The figure shows three views and two pictorial views of one solid part (mm, origin at its lowest corner). Answer the questions. A direction names the side the tool comes from. Give positions to 0.01 mm unless a question says otherwise; leave off trailing zeros. Write each loop counter-clockwise with the first axis right and the second up, starting at its lowest first coordinate (ties: lowest second). Pieces come first, ordered by that corner, then holes. Notation, with made-up numbers: (36, 45.5) -> (54, 45.5) arc R25 cw to (54, 58.5) -> close; hole circle Ø5 at (19, 7). An arc over 180 degrees is marked (long way). Write each question's results on one line, items separated by ' | '. Start each with the question number.
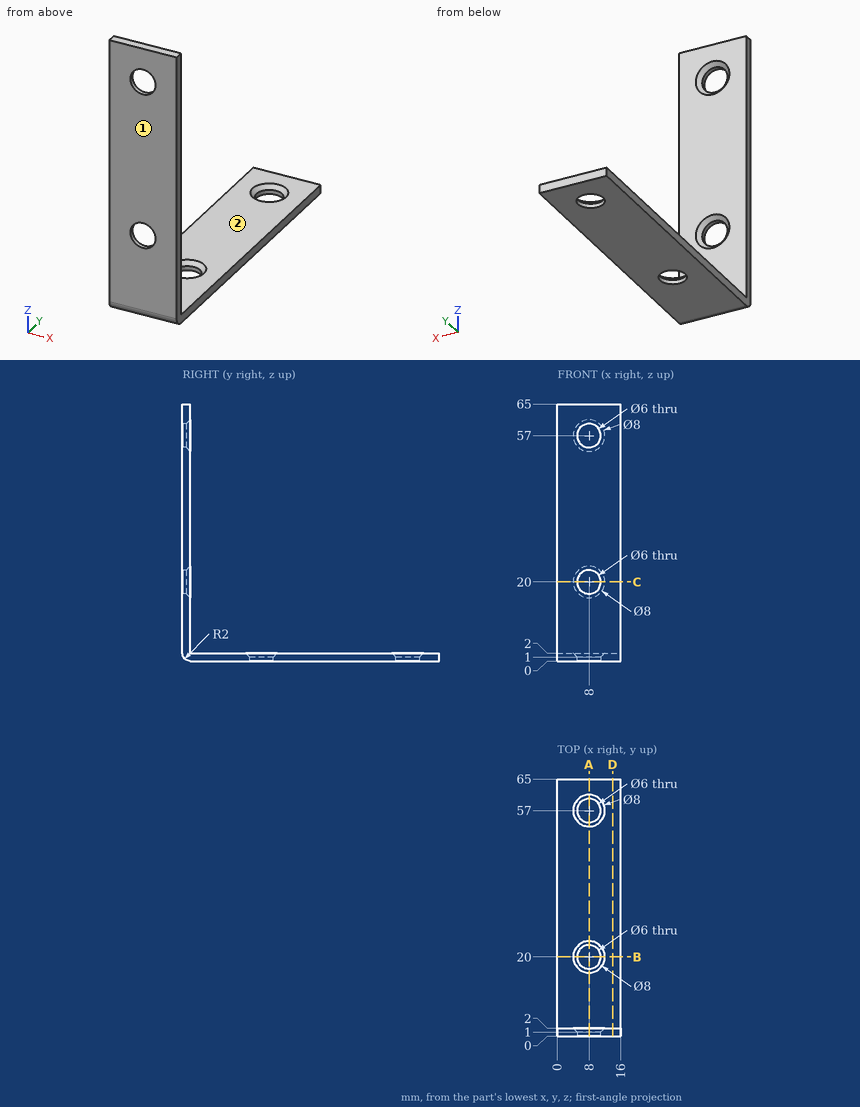
1. Section A-A (x = 8) is taken. Give the number of separate pieces and of enclosed holes in the cut face, then the cut area to 3 significant figures.
2. Section D-D (x = 14) is taken. Write down the section's boundary in (y, z).
3. A tool of negligible diameter and unlimited length cuts with its end or side. For the marked faces 1 and 2, from which of +Z, -Z, +X, -X, +Y, -Y can it reach the whole face along a straight path? Write none if from no direction.
4. Consider probe 1 along Y at (x, z) = (8, 0.6); probe 2 along Z at (x, y) = (8, 0.4); probe 3 along Y at (x, z) = (10.75, 61.5). Determine where each line is inside the solid, lowest interval first. Write a range as [from, to].
5. Each of these flat-tipped pins is pushed along its axis until it touches: pin 1 Ø8 at (x, y) = (6.5, 47) entering from +Z; pin 2 Ø9.5 at (x, z) = (8, 20) entering from +Y; pin 3 Ø5 at (x, z) = (8, 57) entering from +Y. Where does it stop, or does it pass through?
6. Section B-B (y = 20) is taken. Write down the section's boundary in (x, z), then the cut area to 3 significant figures.
Results:
1) separate pieces: 5 | enclosed holes: 0 | area: 203 mm²
2) outline: (0, 2) arc R2 ccw to (2, 0) -> (65, 0) -> (65, 2) -> (2, 2) -> (2, 65) -> (0, 65) -> close
3) face 1: +Z, -Z, +X, -X, -Y | face 2: +Z, +X, -X, +Y
4) probe 1: y = [0.57, 17], [23, 54], [60, 65] | probe 2: z = [0.8, 17], [23, 54], [60, 65] | probe 3: y = [0, 2]
5) pin 1: stops at z = 2 | pin 2: stops at y = 2 | pin 3: passes through
6) outline: (0, 0) -> (5, 0) -> (5, 1) -> (4, 2) -> (0, 2) -> close; (11, 0) -> (16, 0) -> (16, 2) -> (12, 2) -> (11, 1) -> close | area: 19.0 mm²
